```python
from build123d import *

# Parameters (mm, degrees)
BOSS_EXTRUDE1_DEPTH = 5
SKETCH2_R           = 2.5
CUT_EXTRUDE1_DEPTH  = 5
SKETCH3_W           = 15
SKETCH3_H           = 89.364916731
CUT_EXTRUDE2_DEPTH  = 5
SKETCH4_R           = 2.5
CUT_EXTRUDE3_DEPTH  = 5


with BuildPart() as part:
    # Sketch1 → Boss-Extrude1 (new body)
    with BuildSketch(Plane.XY):
        with BuildLine():
            Line((-60, -50), (60, -50))
            ThreePointArc((60, -50), (67.071067812, -47.071067812), (70, -40))
            Line((70, -40), (70, 30))
            ThreePointArc((70, 30), (64.142135624, 44.142135624), (50, 50))
            Line((50, 50), (-50, 50))
            ThreePointArc((-50, 50), (-64.142135624, 44.142135624), (-70, 30))
            Line((-70, 30), (-70, -40))
            ThreePointArc((-70, -40), (-67.071067812, -47.071067812), (-60, -50))
        make_face()
    extrude(amount=BOSS_EXTRUDE1_DEPTH)

    # Sketch2 → Cut-Extrude1 (cut)
    with BuildSketch(Plane.XY.offset(5)):
        with Locations((0, -40)):
            Circle(SKETCH2_R)
        with Locations((-45, 30)):
            Circle(SKETCH2_R)
        with Locations(Location((45, 30, 0), (0, 0, 180))):
            Circle(SKETCH2_R)
        with Locations(Location((-45, -30, 0), (0, 0, 180))):
            Circle(SKETCH2_R)
        with Locations((45, -30)):
            Circle(SKETCH2_R)
    extrude(amount=-CUT_EXTRUDE1_DEPTH, mode=Mode.SUBTRACT)

    # Sketch3 → Cut-Extrude2 (cut)
    with BuildSketch(Plane.XY.offset(5)):
        with Locations((62.5, 4.682458366)):
            Rectangle(SKETCH3_W, SKETCH3_H)
        with Locations((-62.5, 4.682458366)):
            Rectangle(SKETCH3_W, SKETCH3_H)
    extrude(amount=-CUT_EXTRUDE2_DEPTH, mode=Mode.SUBTRACT)

    # Sketch4 → Cut-Extrude3 (cut)
    with BuildSketch(Plane.XY.offset(5)):
        with Locations((0, 20)):
            Circle(SKETCH4_R)
    extrude(amount=-CUT_EXTRUDE3_DEPTH, mode=Mode.SUBTRACT)


solid = part.part
```
Could you check a few things on this model? Use its own coordinates, in mm. A direction names the side the tool comes from. Round coordinates to 2 decimals unless told otherwise and drop trailing zeros. Write each loop counter-clockwise with the first axis right and the second up, starting at its lowest first coordinate (ties: lowest second). Pieces come first, ordered by that corner, then holes.
(1) Thinking about a two-plate mould opening in Y: for faces 1 (the face through (-1, 1, 5)), 2 (the face through (-63, -40, 3)), 3 (the face through (-43.66, 32.11, 2.54)), which applies, +Y half, -Y half, draft (parallel to the pull), parting line (faces both ways), or undercut?
Findings below:
face 1: draft
face 2: +Y half
face 3: undercut
(2) Suppose I cut it at A-A on y = 20. Write out the boundary of the cut face in (x, z), and give its area (3 significant figures).
Findings below:
outline: (-55, 0) - (-2.5, 0) - (-2.5, 5) - (-55, 5) - close; (2.5, 0) - (55, 0) - (55, 5) - (2.5, 5) - close
area: 525 mm2
(3) Suppose I cut it at B-B on x = 45. Write out the boundary of the cut face in (y, z), and give its area (3 significant figures).
Findings below:
outline: (-50, 0) - (-32.5, 0) - (-32.5, 5) - (-50, 5) - close; (-27.5, 0) - (27.5, 0) - (27.5, 5) - (-27.5, 5) - close; (32.5, 0) - (50, 0) - (50, 5) - (32.5, 5) - close
area: 450 mm2
(4) If I drill on probe 1 along Y at (x, z) = (0, 3.6); probe 2 along Y at (x, z) = (-45, 1.95); probe 3 along X at (y, z) = (-13.5, 0.35), over which ranges is the centre line in solid material (lowest first)?
Findings below:
probe 1: y = -50 to -42.5, -37.5 to 17.5, 22.5 to 50
probe 2: y = -50 to -32.5, -27.5 to 27.5, 32.5 to 50
probe 3: x = -55 to 55
(5) Which directions (+Z, -Z, +X, -X, +Y, -Y) give clear straight access to the entire face, cutting with the end or side of a thin tool? Please do faces 4 (the face through (-1, 1, 0)), 5 (the face through (55, 4, 3)), 6 (the face through (-55, 4, 3)).
Findings below:
face 4: -Z, +X, -X, +Y, -Y
face 5: +Z, -Z, +X, +Y
face 6: +Z, -Z, -X, +Y
(6) For pin 1 (12 mm diameter, centred on x = 46, y = -3.5, fed in from -Z); pin 2 (3 mm diameter, centred on x = 0, y = -40, fed in from -Z); pin 3 (1 mm diameter, centred on x = 51.5, z = 0.5, fed in from +Y) (3 decimals); pin 4 (1.5 mm diameter, centred on y = -7.5, z = 2.5, fed in from -X), each with a flat end and sliding along its axis, tell me the tip position at first contact or that it passes through.
Findings below:
pin 1: stops at z = 0
pin 2: passes through
pin 3: stops at y = 49.975
pin 4: stops at x = -55
(7) Suppose I cut it at D-D on y = 30. Write out the boundary of the cut face in (x, z), and give its area (3 significant figures).
Findings below:
outline: (-55, 0) - (-47.5, 0) - (-47.5, 5) - (-55, 5) - close; (-42.5, 0) - (42.5, 0) - (42.5, 5) - (-42.5, 5) - close; (47.5, 0) - (55, 0) - (55, 5) - (47.5, 5) - close
area: 500 mm2
(8) Suppose I cut it at C-C on z = 3.8. Write out the boundary of the cut face in (x, y), and give its area (3 significant figures).
Findings below:
outline: (-70, -40) arc R10 ccw to (-60, -50) - (60, -50) arc R10 ccw to (70, -40) - (55, -40) - (55, 49.36) arc R20 ccw to (50, 50) - (-50, 50) arc R20 ccw to (-55, 49.36) - (-55, -40) - close; hole circle Ø5 at (-45, -30); hole circle Ø5 at (-45, 30); hole circle Ø5 at (0, -40); hole circle Ø5 at (0, 20); hole circle Ø5 at (45, -30); hole circle Ø5 at (45, 30)
area: 11,100 mm2
